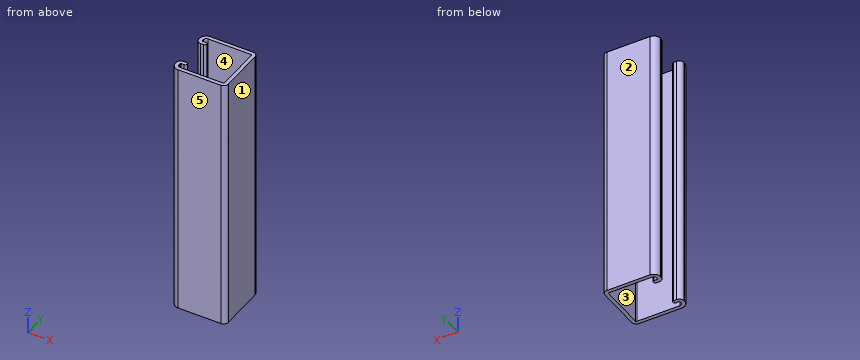
from build123d import *

# Parameters (mm, degrees)
BOSS_EXTRUDE1_DEPTH = 98.425


with BuildPart() as part:
    # Sketch1 → Boss-Extrude1 (new, symmetric)
    with BuildSketch(Plane.XY):
        with BuildLine():
            Line((-36.22675, 20.6375), (-3.46075, 20.6375))
            ThreePointArc((-3.46075, 20.6375), (-1.013630207, 19.623869793), (0, 17.17675))
            Line((0, 17.17675), (0, -17.17675))
            ThreePointArc((0, -17.17675), (-1.013630207, -19.623869793), (-3.46075, -20.6375))
            Line((-3.46075, -20.6375), (-36.22675, -20.6375))
            ThreePointArc((-36.22675, -20.6375), (-39.796401808, -19.158901808), (-41.275, -15.58925))
            Line((-41.275, -15.58925), (-41.275, -14.57325))
            ThreePointArc((-41.275, -14.57325), (-40.261369793, -12.126130207), (-37.81425, -11.1125))
            Line((-37.81425, -11.1125), (-35.5346, -11.1125))
            ThreePointArc((-35.5346, -11.1125), (-34.1376, -12.5095), (-35.5346, -13.9065))
            Line((-35.5346, -13.9065), (-37.81425, -13.9065))
            ThreePointArc((-37.81425, -13.9065), (-38.285713446, -14.101786554), (-38.481, -14.57325))
            Line((-38.481, -14.57325), (-38.481, -15.58925))
            ThreePointArc((-38.481, -15.58925), (-37.820745461, -17.183245461), (-36.22675, -17.8435))
            Line((-36.22675, -17.8435), (-3.46075, -17.8435))
            ThreePointArc((-3.46075, -17.8435), (-2.989286554, -17.648213446), (-2.794, -17.17675))
            Line((-2.794, -17.17675), (-2.794, 17.17675))
            ThreePointArc((-2.794, 17.17675), (-2.989286554, 17.648213446), (-3.46075, 17.8435))
            Line((-3.46075, 17.8435), (-36.22675, 17.8435))
            ThreePointArc((-36.22675, 17.8435), (-37.820745461, 17.183245461), (-38.481, 15.58925))
            Line((-38.481, 15.58925), (-38.481, 14.57325))
            ThreePointArc((-38.481, 14.57325), (-38.285713446, 14.101786554), (-37.81425, 13.9065))
            Line((-37.81425, 13.9065), (-35.5346, 13.9065))
            ThreePointArc((-35.5346, 13.9065), (-34.1376, 12.5095), (-35.5346, 11.1125))
            Line((-35.5346, 11.1125), (-37.81425, 11.1125))
            ThreePointArc((-37.81425, 11.1125), (-40.261369793, 12.126130207), (-41.275, 14.57325))
            Line((-41.275, 14.57325), (-41.275, 15.58925))
            ThreePointArc((-41.275, 15.58925), (-39.796401808, 19.158901808), (-36.22675, 20.6375))
        make_face()
    extrude(amount=BOSS_EXTRUDE1_DEPTH, both=True)


solid = part.part
CAD build for the part. Positions are in the model's coordinates, mm. Face numbers are marked on the shaded views. A direction names the side the tool comes from. Coordinates: 2 decimals unless noted, no trailing zeros. Order: outer loops, then holes, each group sorted by start corner. A loop starts at its lowest first (then second) coordinate and runs counter-clockwise, first axis right, second up. Notation, with made-up numbers: (-34, 69.5) -> (5, 69.5) arc R19 ccw to (5, 82.5) -> close; hole circle Ø2 at (-32.75, 47.25). An arc over 180 degrees is marked (long way). Answer in a Markdown table with one row per item.
1) Which spindle directions (+Z, -Z, +X, -X, +Y, -Y) get a long thin tool onto all of the face, cutting with end or side? Do the marked faces 4 and 5. Say none if no direction does.
Check values:
| item | result |
|---|---|
| face 4 | +Z, -Z |
| face 5 | +Z, -Z, +X, -X, -Y |
2) Band-saw the part on A-A (x = -7.5). List the corners of the cut face in (y, z) (1 decimal).
Check values:
| item | result |
|---|---|
| outline | (-20.6, -98.4) -> (-17.8, -98.4) -> (-17.8, 98.4) -> (-20.6, 98.4) -> close; (17.8, -98.4) -> (20.6, -98.4) -> (20.6, 98.4) -> (17.8, 98.4) -> close |
3) Band-saw the part on C-C (y = -3.5). List the corners of the cut face in (x, z) (3 decimals), and give its area (3 significant figures).
Check values:
| item | result |
|---|---|
| outline | (-2.794, -98.425) -> (0, -98.425) -> (0, 98.425) -> (-2.794, 98.425) -> close |
| area | 550 mm2 |
4) Drill centre lines: line 1 (Y direction, x = -16, z = -82.5); line 2 (X direction, y = -15, z = 88) (3 decimals); line 3 (X direction, y = 9, z = 81.5). Where is each one in solid material? Low to high.
Check values:
| item | result |
|---|---|
| line 1 | -20.64 to -17.84, 17.84 to 20.64 |
| line 2 | -41.275 to -38.481, -2.794 to 0 |
| line 3 | -2.79 to 0 |
5) Mould opens along X. For the marked faces 1, 2 and 3 say: pulls with the +X half, pulls with the -X half, needs draft (parallel to the pull), parting line crosses it, or undercut.
Check values:
| item | result |
|---|---|
| face 1 | pulls with the +X half |
| face 2 | needs draft |
| face 3 | undercut |
6) Flat gauge pins, fed straight in: P1, Ø0.7, axis at x = -36.5, z = 39, coming from the +Y side; P2, Ø17, axis at y = -2, z = -40, coming from the -X side; P3, Ø10, axis at y = -6.5, z = -77.5, coming from the -X side. Where does each tip first touch, or does it go through?
Check values:
| item | result |
|---|---|
| P1 | y = 20.64 |
| P2 | x = -2.79 |
| P3 | x = -39.41 |
7) Band-saw the part on B-B (z = -63). List the corners of the cut face in (x, y) (1 decimal).
Check values:
| item | result |
|---|---|
| outline | (-41.3, -15.6) arc R5 ccw to (-36.2, -20.6) -> (-3.5, -20.6) arc R3.5 ccw to (0, -17.2) -> (0, 17.2) arc R3.5 ccw to (-3.5, 20.6) -> (-36.2, 20.6) arc R5 ccw to (-41.3, 15.6) -> (-41.3, 14.6) arc R3.5 ccw to (-37.8, 11.1) -> (-35.5, 11.1) arc R1.4 ccw to (-35.5, 13.9) -> (-37.8, 13.9) arc R0.7 cw to (-38.5, 14.6) -> (-38.5, 15.6) arc R2.3 cw to (-36.2, 17.8) -> (-3.5, 17.8) arc R0.7 cw to (-2.8, 17.2) -> (-2.8, -17.2) arc R0.7 cw to (-3.5, -17.8) -> (-36.2, -17.8) arc R2.3 cw to (-38.5, -15.6) -> (-38.5, -14.6) arc R0.7 cw to (-37.8, -13.9) -> (-35.5, -13.9) arc R1.4 ccw to (-35.5, -11.1) -> (-37.8, -11.1) arc R3.5 ccw to (-41.3, -14.6) -> close |
